Source: CAD feature listing. Evaluate the final solid. Frame: model axes, mm. A direction names the side the tool comes from. Round coordinates to 2 decimals unless told otherwise and drop trailing zeros. Order: outer loops, then holes, each group sorted by start corner. A loop starts at its lowest first (then second) coordinate and runs counter-clockwise, first axis right, second up. Notation, with made-up numbers: (20, 41.5) -> (27, 41.5) arc R22 ccw to (27, 67.5) -> close; hole circle Ø11 at (-34, 30). An arc over 180 degrees is marked (long way). Write item = value, one per line. Start each with the question number.
(1) Cut plane A-A on x = 25. Return the cut outline in (y, z).
(2) Contact query for flat-ended pins moving along their axis: pin 1 Ø2 at (y, z) = (1, -14) entering from -X; pin 2 Ø4 at (x, y) = (74.5, 11.5) entering from +Z; pin 3 Ø11.5 at (y, z) = (8.5, 6.5) entering from +X; pin 4 Ø1 at (y, z) = (11.5, 1) entering from +X. Output: stop coordinate, or through.
(3) Reachability of faces 1 (the face through (144.013, 17.084, -3.794)), 2 (the face through (268.407, 0, 0)) from +Z, -Z, +X, -X, +Y, -Y: full face, straight path, thin tool, end or side. Return the list, or none.
(4) Cut plane B-B on x = 83.5. Return the cut outline in (y, z).
(5) Ray query, line 1 (Z direction, x = 54, y = -1.5); line 2 (Z direction, x = 40, y = 1); line 3 (X direction, y = 17.5, z = -4). Return the intervals inside material, ascending.
from build123d import *

# Parameters (mm, degrees)
SKETCH1_W = 191.470180192
SKETCH1_H = 17.5


with BuildPart() as part:
    # Sketch1 → Revolve4 (revolve)
    with BuildSketch(Plane.XY, mode=Mode.PRIVATE) as revolve4_sk:
        Polygon((-14.631119083, 30), (-66.59264331, 0), (-14.631119083, 0), align=None)
        Polygon((4.937176498, 30), (-14.631119083, 30), (-14.631119083, 0), (4.937176498, 0), (4.937176498, 19), align=None)
        Polygon((4.937176498, 19), (4.937176498, 0), (46.937176498, 0), (46.937176498, 17.5), (46.937176498, 19), align=None)
        with Locations((142.672266594, 8.75)):
            Rectangle(SKETCH1_W, SKETCH1_H)
        with BuildLine():
            Line((238.40735669, 17.5), (238.40735669, 0))
            Line((238.40735669, 0), (268.40735669, 0))
            Line((268.40735669, 0), (268.40735669, 8))
            Line((268.40735669, 8), (253.40735669, 8))
            Line((253.40735669, 8), (253.40735669, 12.5))
            ThreePointArc((253.40735669, 12.5), (245.501662539, 13.782917549), (238.40735669, 17.5))
        make_face()
    revolve(revolve4_sk.sketch.rotate(Axis((-83.378075763, 0, 0), (1, 0, 0)), 90), axis=Axis((-83.378075763, 0, 0), (1, 0, 0)))


solid = part.part
Evaluation:
q1.outline = circle Ø38 at (0, 0)
q2.pin_1 = -44.01
q2.pin_2 = 14.7
q2.pin_3 = 268.41
q2.pin_4 = 253.41
q3.face_1 = +X
q3.face_2 = +Z, -Z, +X, +Y, -Y
q4.outline = circle Ø35 at (0, 0)
q5.line_1 = -17.44 to 17.44
q5.line_2 = -18.97 to 18.97
q5.line_3 = -35.5 to 46.94
